```python
from build123d import *

# Parameters (mm, degrees)
F1_DEPTH = 16.51
F2_R     = 3.175
F3_DEPTH = 20.574
F4_R     = 4.7625
F5_DEPTH = 7.874
F6_R     = 6.35


with BuildPart() as f1:
    # F0 (on Top) → F1 (new body)
    with BuildSketch(Plane.XY):
        with BuildLine():
            Line((14.859, -48.006), (26.972211, -8.209839))
            ThreePointArc((26.972211, -8.209839), (0, 28.194), (-26.972211, -8.209839))
            Line((-26.972211, -8.209839), (-14.859, -48.006))
            Line((-14.859, -48.006), (14.859, -48.006))
        make_face()
    extrude(amount=F1_DEPTH)

    # F2 (on face) → F3 (join)
    with BuildSketch(Plane.XY.offset(16.51)):
        Circle(F2_R)
    extrude(amount=F3_DEPTH)

    # F4 (on face) → F5 (join)
    with BuildSketch(Plane.XY.offset(16.51)):
        Circle(F4_R)
    extrude(amount=F5_DEPTH)

    # F6
    f6_edges = [f1.edges().sort_by_distance(p)[0] for p in [
        (-14.859, -48.006, 8.255),
        (14.859, -48.006, 8.255),
    ]]
    fillet(f6_edges, radius=F6_R)


solid = f1.part
```
Geometry: final body of the model. Coordinates: model frame, mm. A direction names the side the tool comes from. Coordinates: 2 decimals unless noted, no trailing zeros. Order: outer loops, then holes, each group sorted by start corner. A loop starts at its lowest first (then second) coordinate and runs counter-clockwise, first axis right, second up. Notation, with made-up numbers: (51, -1.5) - (57, -1.5) arc R21 ccw to (57, 2.5) - close; hole circle Ø1 at (38, -12). An arc over 180 degrees is marked (long way). Write each question's results on one line, items separated by ' | '.
1) Section C-C, the plane z = 5.5. Return loops of the section in (x, y), plus the area to 3 significant figures.
Results list:
outline: (-26.97, -8.21) - (-16.23, -43.51) arc R6.35 ccw to (-10.15, -48.01) - (10.15, -48.01) arc R6.35 ccw to (16.23, -43.51) - (26.97, -8.21) arc R28.19 ccw (long way) to start | area: 3,360 mm^2
2) Section A-A, the plane y = 0. Return loops of the section in (x, z) (1 decimal), plus the area to 3 significant figures.
Results list:
outline: (-28.2, 0) - (28.2, 0) - (28.2, 16.5) - (4.8, 16.5) - (4.8, 24.4) - (3.2, 24.4) - (3.2, 37.1) - (-3.2, 37.1) - (-3.2, 24.4) - (-4.8, 24.4) - (-4.8, 16.5) - (-28.2, 16.5) - close | area: 1,090 mm^2
3) Section D-D, the plane z = 18. Return loops of the section in (x, y) (1 decimal).
Results list:
outline: circle Ø9.5 at (0, 0)
4) Line query: line 1 (Z direction, x = -14, y = -41.5); line 2 (Y direction, x = -0.5, z = 4.5); line 3 (Y direction, x = 10.5, z = 4). Output: solid intervals per line, ascending. Write a range as from..to.
Results list:
line 1: 0..16.51 | line 2: -48.01..28.19 | line 3: -48..26.17
5) Set-up query: faces 1 (the cylindrical face through (0.737, 28.184, 8.139)), 2 (the cylindrical face through (-3.78, -2.9, 20.39)). Return all of +Z, -Z, +X, -X, +Y, -Y with unobstructed straight access to the full face (end or side cutting, diameter ignored); none if empty.
Results list:
face 1: +Z, -Z | face 2: +Z
6) Pin query (flat end, axial travel): pin 1 (1 mm diameter, centred on x = 3, y = -33, fed in from +Z); pin 2 (2 mm diameter, centred on x = 4.5, z = 27.5, fed in from -Y); pin 3 (10 mm diameter, centred on x = 12.5, z = 18.5, fed in from +Y); pin 4 (8 mm diameter, centred on x = 19.5, z = 5, fed in from -Y). Return the tip coordinate at first contact, or that it passes through.
Results list:
pin 1: z = 16.51 | pin 2: through | pin 3: y = 27.06 | pin 4: y = -45.08
7) Section B-B, the plane x = 0. Return loops of the section in (y, z) (1 decimal), plus the area to 3 significant figures.
Results list:
outline: (-48, 0) - (28.2, 0) - (28.2, 16.5) - (4.8, 16.5) - (4.8, 24.4) - (3.2, 24.4) - (3.2, 37.1) - (-3.2, 37.1) - (-3.2, 24.4) - (-4.8, 24.4) - (-4.8, 16.5) - (-48, 16.5) - close | area: 1,410 mm^2
